```python
from build123d import *

# Parameters (mm, degrees)
CROQUIS1_R              = 2
CROQUIS1_R_2            = 1.5
SALIENTE_EXTRUIR1_DEPTH = 1
REDONDEO1_R             = 3
SCALE1_SCALE            = 0.888889
SKETCH1_R               = 1.5
BOSS_EXTRUDE1_DEPTH     = 1.777778
BOSS_EXTRUDE2_DEPTH     = 1.777778
SKETCH3_R               = 4.6
CUT_EXTRUDE1_DEPTH      = 10
SKETCH4_R               = 2
SKETCH4_R_2             = 1.5
BOSS_EXTRUDE3_DEPTH     = 12


with BuildPart() as part:
    # Croquis1 → Saliente-Extruir1 (new, symmetric)
    with BuildSketch(Plane(origin=(0, 0, 0), x_dir=(1, 0, 0), z_dir=(0, 1, 0))):
        Polygon((12.846621, 7), (17.5, 17.599716), (17.5, 47.599716), (8, 62), (-8, 62), (-17.5, 47.599716), (-17.5, 17.599716), (-12.846621, 7), align=None)
        with Locations(Location((0, 21, 0), (0, 0, 270))):
            Circle(CROQUIS1_R, mode=Mode.SUBTRACT)
        with Locations(Location((-5.25, 57.994262, 0), (0, 0, 270))):
            Circle(CROQUIS1_R_2, mode=Mode.SUBTRACT)
        with Locations(Location((-13.5, 37.599716, 0), (0, 0, 270))):
            Circle(CROQUIS1_R_2, mode=Mode.SUBTRACT)
        with Locations(Location((13.5, 37.599716, 0), (0, 0, 270))):
            Circle(CROQUIS1_R_2, mode=Mode.SUBTRACT)
        with Locations(Location((5.25, 57.994262, 0), (0, 0, 270))):
            Circle(CROQUIS1_R_2, mode=Mode.SUBTRACT)
        with Locations(Location((-6, 11, 0), (0, 0, 270))):
            Circle(CROQUIS1_R_2, mode=Mode.SUBTRACT)
        with Locations(Location((6, 11, 0), (0, 0, 270))):
            Circle(CROQUIS1_R_2, mode=Mode.SUBTRACT)
    extrude(amount=SALIENTE_EXTRUIR1_DEPTH, both=True)

    # Redondeo1
    redondeo1_edges = [part.edges().sort_by_distance(p)[0] for p in [
        (17.5, 0, -17.599716),
        (-17.5, 0, -17.599716),
        (-17.5, 0, -47.599716),
        (-8, 0, -62),
        (8, 0, -62),
        (17.5, 0, -47.599716),
    ]]
    fillet(redondeo1_edges, radius=REDONDEO1_R)


with BuildPart() as part_1:
    # Scale1: scaled about (0, 0, -33.418377)
    add(part.part.scale(SCALE1_SCALE).moved(Location((0, 0, -3.713153))))

    # Sketch1 → Boss-Extrude1 (add)
    with BuildSketch(Plane.XZ.offset(0.888889)):
        with BuildLine():
            Line((-15.555556, -31.135123), (-46.555556, -31.135123))
            ThreePointArc((-46.555556, -31.135123), (-47.969769, -31.720909), (-48.555556, -33.135123))
            Line((-48.555556, -33.135123), (-48.555556, -41.135123))
            ThreePointArc((-48.555556, -41.135123), (-47.969769, -42.549336), (-46.555556, -43.135123))
            Line((-46.555556, -43.135123), (-15.555556, -43.135123))
            Line((-15.555556, -43.135123), (-15.555556, -39.635123))
            Line((-15.555556, -39.635123), (-44.013891, -39.635123))
            ThreePointArc((-44.013891, -39.635123), (-44.367444, -39.488676), (-44.513891, -39.135123))
            Line((-44.513891, -39.135123), (-44.513891, -35.135123))
            ThreePointArc((-44.513891, -35.135123), (-44.367444, -34.781569), (-44.013891, -34.635123))
            Line((-44.013891, -34.635123), (-15.555556, -34.635123))
            Line((-15.555556, -34.635123), (-15.555556, -31.135123))
        make_face()
        with Locations(Location((-46.5, -33.135123, 0), (0, 0, 270))):
            Circle(SKETCH1_R, mode=Mode.SUBTRACT)
        with Locations(Location((-46.5, -41.135123, 0), (0, 0, 270))):
            Circle(SKETCH1_R, mode=Mode.SUBTRACT)
    extrude(amount=-BOSS_EXTRUDE1_DEPTH)

    # Sketch2 → Boss-Extrude2 (add)
    with BuildSketch(Plane(origin=(0, 0.888889, 0), x_dir=(1, 0, 0), z_dir=(0, 1, 0))):
        with BuildLine():
            Line((-16.898979, 39.635123), (-15.555556, 39.635123))
            Line((-15.555556, 39.635123), (-15.555556, 34.635123))
            Line((-15.555556, 34.635123), (-17.00037, 34.635123))
            ThreePointArc((-17.00037, 34.635123), (-17.545203, 37.147199), (-16.898979, 39.635123))
        make_face()
    extrude(amount=-BOSS_EXTRUDE2_DEPTH)

    # Sketch3 → Cut-Extrude1 (cut)
    with BuildSketch(Plane(origin=(0, 0.888889, 0), x_dir=(1, 0, 0), z_dir=(0, 1, 0))):
        with Locations(Location((-12, 37.135123, 0), (0, 0, 270))):
            Circle(SKETCH3_R)
    extrude(amount=-CUT_EXTRUDE1_DEPTH, mode=Mode.SUBTRACT)

    # Sketch4 → Boss-Extrude3 (add)
    # profile 1 of 2: a face of its own
    with BuildSketch(Plane(origin=(0, 0.888889, 0), x_dir=(1, 0, 0), z_dir=(0, 1, 0))):
        with Locations(Location((-46.555556, 41.135123, 0), (0, 0, 90))):
            Circle(SKETCH4_R)
        with Locations(Location((-46.5, 41.135123, 0), (0, 0, 90))):
            Circle(SKETCH4_R_2, mode=Mode.SUBTRACT)
    # profile 2 of 2: a face of its own
    with BuildSketch(Plane(origin=(0, 0.888889, 0), x_dir=(1, 0, 0), z_dir=(0, 1, 0))):
        with Locations(Location((-46.555556, 33.135123, 0), (0, 0, 270))):
            Circle(SKETCH4_R)
        with Locations(Location((-46.5, 33.135123, 0), (0, 0, 90))):
            Circle(SKETCH4_R_2, mode=Mode.SUBTRACT)
    extrude(amount=BOSS_EXTRUDE3_DEPTH)


solid = part_1.part
```
Model file for the job. Use its own axes, mm. A direction names the side the tool comes from. Coordinates: 2 decimals unless noted, no trailing zeros. Order: outer loops, then holes, each group sorted by start corner. A loop starts at its lowest first (then second) coordinate and runs counter-clockwise, first axis right, second up. Notation, with made-up numbers: (-6, 15) - (42, 15) arc R15 cw to (42, 24) - close; hole circle Ø9 at (3.5, 12). An arc over 180 degrees is marked (long way). Return JSON: item names as keys, results as strings. Group by question number.
1) Saw through at A-A, the plane x = 0. Write the cut outline in (y, z), plus the area to 3 significant figures.
2) Saw through at B-B, the plane y = 4.5. Write the cut outline in (x, z).
3) Flat gauge pins, fed straight in: P1, Ø5, axis at x = -28, z = -42.5, coming from the +Y side; P2, Ø1.4, axis at x = -31.5, y = -0.5, coming from the -Z side; P3, Ø1.4, axis at y = 0, z = -43.5, coming from the -X side; P4, Ø5, axis at x = -46.5, z = -41.14, coming from the -Y side. Where does each tip first touch, or does it go through?
4) Saw through at C-C, the plane x = -13.5. Write the cut outline in (y, z), plus the area to 3 significant figures.
5) Tool access for faces 5 (the flat face through (-31, 0, -43.135)), 6 (the cylindrical face through (-47.16, 6.8, -43.04)), 7 (the flat face through (0, 0, -9.935)), 8 (the flat face through (-15.556, 0, -26)), 9 (the flat face through (-31, 0, -34.635)): list every direction of +Z, -Z, +X, -X, +Y, -Y with a clear straight run to the whole face (end or side of a thin tool).
6) Probe line 1 (Z direction, x = -46.5, y = 4.5); line 2 (Z direction, x = -5, y = 0.5); line 3 (Z direction, x = -33.5, y = -0.5). List the from-to ranges inside material, lowest first. Write a range as from..to.
7) Mould opens along X. For faces 1 (the cylindrical face through (4.82, -0.01, -12.26)), 2 (the flat face through (-44.514, 0, -37)), 3 (the cylindrical face through (-6.956, 0.012, -58.497)), 4 (the flat face through (11.56, 0.01, -52.08)) say: released by +X, released by -X, zero draft, split by the parting line, or undercut.
Values found:
{
 "1": {"outline": "(-0.89, -58.82) - (0.89, -58.82) - (0.89, -24.16) - (-0.89, -24.16) - close; (-0.89, -20.6) - (0.89, -20.6) - (0.89, -9.94) - (-0.89, -9.94) - close", "area": "80.6 mm²"},
 "2": {"outline": "circle Ø4 at (-46.56, -41.14); circle Ø4 at (-46.56, -33.14); hole circle Ø3 at (-46.5, -41.14); hole circle Ø3 at (-46.5, -33.14)"},
 "3": {"P1": "stops at y = 0.89", "P2": "stops at z = -43.14", "P3": "stops at x = -47.66", "P4": "stops at y = -0.89"},
 "4": {"outline": "(-0.89, -49.14) - (0.89, -49.14) - (0.89, -41.48) - (-0.89, -41.48) - close; (-0.89, -32.79) - (0.89, -32.79) - (0.89, -14.68) - (-0.89, -14.68) - close", "area": "45.8 mm²"},
 "5": {"face 5": "-Z, -X, +Y, -Y", "face 6": "+Y", "face 7": "+Z, +X, -X, +Y, -Y", "face 8": "+Z, -X, +Y, -Y", "face 9": "+Y, -Y"},
 "6": {"line 1": "z = -43.13..-42.64, -39.64..-39.14, -35.13..-34.64, -31.64..-31.14", "line 2": "z = -58.82..-56.55, -53.97..-14.78, -12.2..-9.94", "line 3": "z = -43.14..-39.64, -34.64..-31.14"},
 "7": {"face 1": "undercut", "face 2": "undercut", "face 3": "released by -X", "face 4": "released by +X"}
}
